Verification items for the finished model (mm, model axes). Face numbers are marked on the shaded views. A direction names the side the tool comes from. Give positions to 0.01 mm unless a question says otherwise; leave off trailing zeros. Write each loop counter-clockwise with the first axis right and the second up, starting at its lowest first coordinate (ties: lowest second). Pieces come first, ordered by that corner, then holes. Notation, with made-up numbers: (15, -1) -> (30, -1) arc R4 ccw to (30, 5) -> close; hole circle Ø4 at (82, -38). An arc over 180 degrees is marked (long way). Write item = value, one per line.
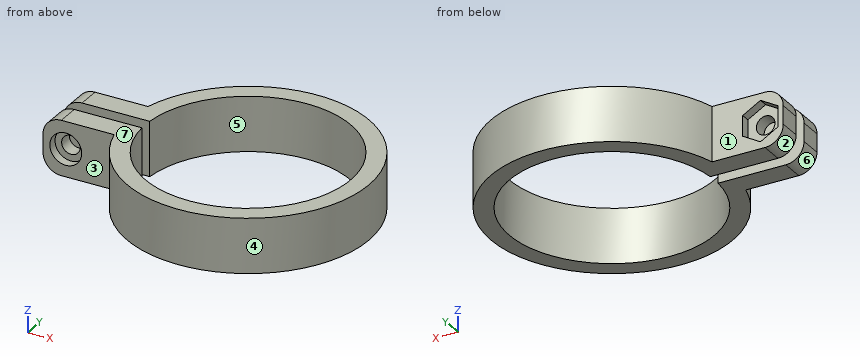
from build123d import *

# Parameters (mm, degrees)
F1_DEPTH = 6
F2_R     = 2.05
F4_DEPTH = 13
F2_R_2   = 3.5
F5_DEPTH = 2
F6_DEPTH = 2
F7_R     = 4


with BuildPart() as f1:
    # F0 (on Top) → F1 (new body, symmetric)
    with BuildSketch(Plane.XY):
        with BuildLine():
            ThreePointArc((-22.449944, 1.5), (22.5, 0), (-22.449944, -1.5))
            Line((-22.449944, -1.5), (-41.327112, -1.5))
            Line((-41.327112, -1.5), (-41.327112, -6.5))
            Line((-41.327112, -6.5), (-25.690465, -6.5))
            ThreePointArc((-25.690465, -6.5), (26.5, 0), (-25.690465, 6.5))
            Line((-25.690465, 6.5), (-41.327112, 6.5))
            Line((-41.327112, 6.5), (-41.327112, 1.5))
            Line((-41.327112, 1.5), (-22.449944, 1.5))
        make_face()
    extrude(amount=F1_DEPTH, both=True)

    # F2 (on face) → F4 (cut, through all)
    with BuildSketch(Plane.XZ.offset(6.5)):
        with Locations((-36.327112, 0)):
            Circle(F2_R)
    extrude(amount=-F4_DEPTH, mode=Mode.SUBTRACT)

    # F2 (on face) → F5 (cut)
    with BuildSketch(Plane.XZ.offset(6.5)):
        with Locations((-36.327112, 0)):
            Circle(F2_R_2)
        with Locations((-36.327112, 0)):
            Circle(F2_R, mode=Mode.SUBTRACT)
    extrude(amount=-F5_DEPTH, mode=Mode.SUBTRACT)

    # F3 (on face) → F6 (cut)
    with BuildSketch(Plane(origin=(0, 6.5, 0), x_dir=(-1, 0, 0), z_dir=(0, 1, 0))):
        Polygon((40.224226, -2.25), (40.224226, 2.25), (36.327112, 4.5), (32.429997, 2.25), (32.429997, -2.25), (36.327112, -4.5), align=None)
    extrude(amount=-F6_DEPTH, mode=Mode.SUBTRACT)

    # F7
    f7_edges = [f1.edges().sort_by_distance(p)[0] for p in [
        (-41.327112, 4, 6),
        (-41.327112, -4, 6),
        (-41.327112, 4, -6),
        (-41.327112, -4, -6),
    ]]
    fillet(f7_edges, radius=F7_R)


solid = f1.part
Item 1: Sectioned sample at B-B on y = 2.5. Record the cut outline in (x, z).
Response values:
outline = (-41.33, -2) arc R4 ccw to (-37.33, -6) -> (-22.36, -6) -> (-22.36, 6) -> (-37.33, 6) arc R4 ccw to (-41.33, 2) -> close; (22.36, -6) -> (26.38, -6) -> (26.38, 6) -> (22.36, 6) -> close; hole circle Ø4.1 at (-36.33, 0)
Item 2: Material ranges on line 1 (Y direction, x = 0.5, z = -2.25); line 2 (Y direction, x = -30.5, z = -1.5); line 3 (X direction, y = 5, z = 1.25), recorded low to high.
Response values:
line_1 = -26.5 to -22.49, 22.49 to 26.5
line_2 = -6.5 to -1.5, 1.5 to 6.5
line_3 = -41.33 to -40.22, -32.43 to -21.94, 21.94 to 26.02
Item 3: Go/stop test with flat-tipped pins: P1, Ø1, axis at y = -12, z = 1.5, coming from the -X side; P2, Ø3.5, axis at x = -37, z = -0.5, coming from the -Y side; P3, Ø3, axis at y = -11, z = -1, coming from the -X side; P4, Ø5, axis at x = -32.5, y = -8, coming from the -Z side. Record where each tip stops, or that it passes through.
Response values:
P1 = -23.87
P2 = -4.5
P3 = -24.74
P4 = -6
Item 4: Sectioned sample at D-D on y = -20.5. Record the cut outline in (x, z).
Response values:
outline = (-16.79, -6) -> (-9.27, -6) -> (-9.27, 6) -> (-16.79, 6) -> close; (9.27, -6) -> (16.79, -6) -> (16.79, 6) -> (9.27, 6) -> close
Item 5: Set-up check for the marked faces 1, 2 and 3: record each of +Z, -Z, +X, -X, +Y, -Y from which the full face is reachable in a straight line by a thin tool's end or side.
Response values:
face_1 = +Z, -Z, -X, +Y
face_2 = -Z, -X, +Y, -Y
face_3 = +Z, -Z, -X, -Y
Item 6: Mould release check, pull along X, two halves, no side actions. Record for the marked faces 4, 5, 6 and 7: +X half, -X half, draft (parallel to the pull), parting line (faces both ways), or undercut.
Response values:
face_4 = parting line
face_5 = undercut
face_6 = -X half
face_7 = draft
Item 7: Sectioned sample at C-C on x = 0. Record the cut outline in (y, z).
Response values:
outline = (-26.5, -6) -> (-22.5, -6) -> (-22.5, 6) -> (-26.5, 6) -> close; (22.5, -6) -> (26.5, -6) -> (26.5, 6) -> (22.5, 6) -> close
Item 8: Sectioned sample at A-A on z = 0. Record the cut outline in (x, y), then the cut area to 3 significant figures.
Response values:
outline = (-41.33, -6.5) -> (-39.83, -6.5) -> (-39.83, -4.5) -> (-38.38, -4.5) -> (-38.38, -1.5) -> (-41.33, -1.5) -> close; (-41.33, 1.5) -> (-38.38, 1.5) -> (-38.38, 4.5) -> (-40.22, 4.5) -> (-40.22, 6.5) -> (-41.33, 6.5) -> close; (-34.28, -4.5) -> (-32.83, -4.5) -> (-32.83, -6.5) -> (-25.69, -6.5) arc R26.5 ccw (long way) to (-25.69, 6.5) -> (-32.43, 6.5) -> (-32.43, 4.5) -> (-34.28, 4.5) -> (-34.28, 1.5) -> (-22.45, 1.5) arc R22.5 cw (long way) to (-22.45, -1.5) -> (-34.28, -1.5) -> close
area = 701 mm^2
